Read the model definition and answer for the solid it produces. Units are mm, in the model's axes. Face numbers are marked on the shaded views. A direction names the side the tool comes from. Round coordinates to 2 decimals unless told otherwise and drop trailing zeros. Order: outer loops, then holes, each group sorted by start corner. A loop starts at its lowest first (then second) coordinate and runs counter-clockwise, first axis right, second up. Notation, with made-up numbers: (-29, 74.5) - (21, 74.5) arc R26 cw to (21, 106.5) - close; hole circle Ø3 at (37.5, 43.25). An arc over 180 degrees is marked (long way). One line per question, with ' | ' between items. Start each with the question number.
1) The part is cut by section A-A, the plane y = 30. Give the vertices of the cut face in (x, z).
2) Straight lines are drawn through the part: line 1 (Z direction, x = 56.5, y = 30); line 2 (X direction, y = 13, z = -1.5); line 3 (X direction, y = 19.5, z = 12.25). For each, find the intervals that lie inside material, in ascending order. Write a range as from..to.
3) For the marked faces 1 and 2, determine the directions among +Z, -Z, +X, -X, +Y, -Y from which every point of the face is accessible in a straight line to the end or side of a thin tool.
4) Flat-ended cylindrical pins translate along their axes: pin 1 (12 mm diameter, centred on x = -26.5, y = 17.5, fed in from +Z); pin 2 (3.5 mm diameter, centred on x = 36, y = 12, fed in from +Z); pin 3 (1 mm diameter, centred on x = 37, y = 14, fed in from -Z); pin 4 (3.5 mm diameter, centred on x = -36.5, z = 5, fed in from +Y). Find the tip coordinate at first contact, or state that the pin passes through.
5) The mould has two halves that part along X. Classify the marked faces 3, 4, 5 and 6: pulls with the +X half, pulls with the -X half, needs draft (parallel to the pull), parting line crosses it, or undercut.
6) The part is cut by section B-B, the plane x = -28. Give the vertices of the cut face in (y, z).
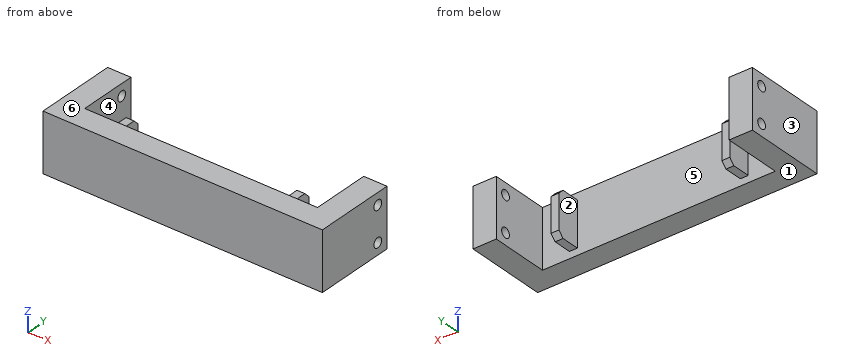
Autodesk Inventor part; units mm, degrees
ref_plane "YZ Plane" through (0, 0, 0) normal (1, 0, 0) x (0, 1, 0)
ref_plane "XZ Plane" through (0, 0, 0) normal (0, 1, 0) x (-1, 0, 0)
ref_plane "XY Plane" through (0, 0, 0) normal (0, 0, 1) x (1, 0, 0)
sketch "Эскиз1" plane through (0, 0, 0) normal (0, 1, 0) x (-1, 0, 0)
  line L0 (50, 15.4) -> (40.5, 15.4)
  line L1 (50, 15.4) -> (-50, 15.4)
  line L2 (-50, -9.6) -> (-50, 15.4)
  line L3 (50, -9.6) -> (40.5, -9.6)
  line L4 (50, -9.6) -> (-50, -9.6)
  line L5 (50, 15.4) -> (-50, 15.4)
  line L6 (-50, 15.4) -> (-50, -9.6)
  line L7 (-50, -9.6) -> (50, -9.6)
  line L8 (50, -9.6) -> (50, 15.4)
  line L9 (38.4, 12.5) -> (38.4, -6.7)
  line L10 (38.4, 12.5) -> (35, 12.5)
  line L11 (35, 12.5) -> (35, -6.7)
  line L12 (35, -6.7) -> (38.4, -6.7)
  line L13 (38.4, -6.7) -> (38.4, 12.5)
  line L14 (-35, -9.6) -> (-35, 15.4)
  line L15 (-35, -9.6) -> (-38.4, -9.6)
  line L16 (-35, 15.4) -> (-38.4, 15.4)
  line L17 (-38.4, 15.4) -> (-38.4, -9.6)
  line L18 (-38.4, -9.6) -> (-35, -9.6)
  line L19 (-35, -9.6) -> (-35, 15.4)
  line L20 (50, 15.4) -> (60, 15.4)
  line L21 (60, 15.4) -> (60, -9.6)
  line L22 (60, -9.6) -> (50, -9.6)
  line L23 (50, -9.6) -> (50, 15.4)
  line L24 (-50, 15.4) -> (-60, 15.4)
  line L25 (-60, 15.4) -> (-60, -9.6)
  line L26 (-60, -9.6) -> (-50, -9.6)
  line L27 (-50, -9.6) -> (-50, 15.4)
  line L28 (-35, -6.7) -> (-38.4, -6.7)
  line L29 (-35, 12.5) -> (-38.4, 12.5)
  point P0 (0, 0)
  point P1 (0, 0)
  point P2 (50, 15.4)
  dimension "d10" = 25
  dimension "d1" = 10
  dimension "d2" = 10
  dimension "d9" = 25
  dimension "d11" = 2.9
  dimension "d12" = 25
  dimension "d13" = 2.9
  dimension "d15" = 2.9
extrude "Выдавливание1" add sketch "Эскиз1" along normal blind 10 contours L8 L3 L4 L14 L1 L0 | L20 L21 L22 L8 | L14 L29 L17 L1 | L17 L4 L2 L1 | L14 L28 L17 L29 | L4 L17 L28 L14 | L2 L26 L25 L24 | L9 L12 L11 L10
sketch "Эскиз2" plane through (0, 10, 0) normal (0, 1, 0) x (1, 0, 0)
  line L0 (-60, 9.6) -> (-60, -15.4)
  line L1 (60, 9.6) -> (-60, 9.6)
  line L2 (-60, -15.4) -> (60, -15.4)
  line L3 (60, -15.4) -> (60, 9.6)
  line L4 (60, 9.6) -> (-60, 9.6)
  line L5 (-60, 9.6) -> (-60, -15.4)
  line L6 (60, -15.4) -> (60, 9.6)
  line L7 (60, -15.4) -> (50, -15.4)
  line L8 (50, -15.4) -> (50, 9.6)
  line L9 (50, 9.6) -> (60, 9.6)
  line L10 (60, 9.6) -> (60, -15.4)
  line L11 (-60, -15.4) -> (60, -15.4)
  line L12 (-60, -15.4) -> (-50, -15.4)
  line L13 (-50, -15.4) -> (-50, 9.6)
  line L14 (-50, 9.6) -> (-60, 9.6)
  line L15 (-60, 9.6) -> (-60, -15.4)
  dimension "d16" = 10
  dimension "d17" = 10
extrude "Выдавливание2" add sketch "Эскиз2" along normal blind 25 contours L1 L13 L2 L0 | L1 L3 L2 L8
sketch "Эскиз3" plane through (60, 0, 15.4) normal (1, 0, 0) x (0, 0, -1)
  line L0 (0, 25) -> (0, 35)
  line L1 (0, 30) -> (25, 30)
  line L2 (25, 25) -> (25, 35)
  circle A0 centre (5, 30) radius 2.1
  circle A1 centre (20, 30) radius 2.1
  line L3 (0, 35) -> (25, 35)
  point P0 (15.4, 0)
  point P1 (50, 0)
  dimension "d18" = 4.2
  dimension "d19" = 4.2
  dimension "d20" = 5
  dimension "d21" = 5
extrude "Выдавливание3" cut sketch "Эскиз3" against normal blind 127.5 contours A0 L1 | L1 A0 | A1 L1 | L1 A1
sketch "Эскиз4" plane through (0, 10, 0) normal (0, 1, 0) x (1, 0, 0)
  line L0 (50, 9.6) -> (40.5, 9.6)
  line L1 (50, 9.6) -> (-50, 9.6)
  line L2 (-50, -15.4) -> (-50, 9.6)
  line L3 (50, -15.4) -> (40.5, -15.4)
  line L4 (50, -15.4) -> (-50, -15.4)
  line L5 (50, 9.6) -> (-50, 9.6)
  line L6 (-50, 9.6) -> (-50, -15.4)
  line L7 (-50, -15.4) -> (50, -15.4)
  line L8 (50, -15.4) -> (50, 9.6)
  line L9 (38.4, 6.7) -> (38.4, -12.5)
  line L10 (38.4, 6.7) -> (35, 6.7)
  line L11 (35, 6.7) -> (35, -12.5)
  line L12 (35, -12.5) -> (38.4, -12.5)
  line L13 (38.4, -12.5) -> (38.4, 6.7)
  line L14 (-35, -15.4) -> (-35, 9.6)
  line L15 (-35, -15.4) -> (-38.4, -15.4)
  line L16 (-35, 9.6) -> (-38.4, 9.6)
  line L17 (-38.4, 9.6) -> (-38.4, -15.4)
  line L18 (-38.4, -15.4) -> (-35, -15.4)
  line L19 (-35, -15.4) -> (-35, 9.6)
  line L20 (50, 9.6) -> (60, 9.6)
  line L21 (60, 9.6) -> (60, -15.4)
  line L22 (60, -15.4) -> (50, -15.4)
  line L23 (50, -15.4) -> (50, 9.6)
  line L24 (-50, 9.6) -> (-60, 9.6)
  line L25 (-60, 9.6) -> (-60, -15.4)
  line L26 (-60, -15.4) -> (-50, -15.4)
  line L27 (-50, -15.4) -> (-50, 9.6)
  line L28 (-35, -12.5) -> (-38.4, -12.5)
  line L29 (-35, 6.7) -> (-38.4, 6.7)
  point P0 (0, 0)
  point P1 (0, 0)
  point P2 (0, 0)
  point P3 (50, 9.6)
  dimension "d27" = 25
  dimension "d24" = 10
  dimension "d25" = 10
  dimension "d26" = 25
  dimension "d28" = 2.9
  dimension "d29" = 25
  dimension "d30" = 2.9
  dimension "d31" = 2.9
extrude "Выдавливание4" add sketch "Эскиз4" along normal blind 10 contours L14 L28 L17 L29 | L9 L12 L11 L10
chamfer "Фаска1" distance 2.25 angle 45 4 edges at (-36.7, 20, 12.5) (-36.7, 20, -6.7) (36.7, 20, 12.5) (36.7, 20, -6.7)
equation "\"d19\" = d18"
equation "\"d20\" = d21"
properties part number "000.201 - Балка несущая"
Values:
1) outline: (-60, -9.6) - (-50, -9.6) - (-50, -6.7) - (-60, -6.7) - close; (-60, -2.5) - (-50, -2.5) - (-50, 8.3) - (-60, 8.3) - close; (-60, 12.5) - (-50, 12.5) - (-50, 15.4) - (-60, 15.4) - close; (50, -9.6) - (60, -9.6) - (60, -6.7) - (50, -6.7) - close; (50, -2.5) - (60, -2.5) - (60, 8.3) - (50, 8.3) - close; (50, 12.5) - (60, 12.5) - (60, 15.4) - (50, 15.4) - close
2) line 1: z = -9.6..-6.7, -2.5..8.3, 12.5..15.4 | line 2: x = -60..-50, -38.4..-35, 35..38.4, 50..60 | line 3: x = -60..-50, 50..60
3) face 1: -Z, +X, -X, +Y, -Y | face 2: +Z, -Z, +Y
4) pin 1: passes through | pin 2: stops at z = 12.5 | pin 3: stops at z = -6.7 | pin 4: stops at y = 20
5) face 3: pulls with the -X half | face 4: undercut | face 5: undercut | face 6: needs draft
6) outline: (0, -9.6) - (10, -9.6) - (10, 15.4) - (0, 15.4) - close
